Geometry: final body of the model. Coordinates: model frame, mm. Give positions to 0.01 mm unless a question says otherwise; leave off trailing zeros. Write each loop counter-clockwise with the first axis right and the second up, starting at its lowest first coordinate (ties: lowest second). Pieces come first, ordered by that corner, then holes. Notation, with made-up numbers: M -17,7 L 32,7 A26 cw 32,36 Z; hole C -37.5,45.25 d7. An arc over 180 degrees is marked long. Use a Markdown table: item, result. Add a question column.
(1) Draft query along Z for faces 1 (the flat face through (11, 25, 127)), 2 (the flat face through (12, 50.8, 2)), 3 (the cylindrical face through (825.44, 25.04, -2.79)). Return one class per face: released by +Z, released by -Z, zero draft, split by the parting line, or undercut.
(2) Cut plane D-D (z = -90.5). Output: boundary loops of the cut face in (x, y).
(3) Material intervals for L1, parallel to X at y = 22, z = -25.5; L2, parallel to Z at x = -762, y = 34; L3, parallel to X at y = 22, z = 51, sorted ascending.
(4) Cut plane B-B (y = 42). Output: boundary loops of the cut face in (x, z).
(5) Cut plane C-C (z = 79). Output: boundary loops of the cut face in (x, y).
(6) Cut plane A-A (z = 0). Output: boundary loops of the cut face in (x, y), plus the area to 3 significant figures.
(7) Pin query (flat end, axial travel): pin 1 Ø3 at (y, z) = (21.5, 93) entering from +X; pin 2 Ø3 at (y, z) = (21, -89) entering from -X; pin 3 Ø4 at (y, z) = (24, -84.5) entering from +X. Return the tip coordinate at first contact, or that it passes through.
Autodesk Inventor part; units mm, degrees
ref_plane "YZ Plane" through (0, 0, 0) normal (1, 0, 0) x (0, 1, 0)
ref_plane "XZ Plane" through (0, 0, 0) normal (0, 1, 0) x (-1, 0, 0)
ref_plane "XY Plane" through (0, 0, 0) normal (0, 0, 1) x (1, 0, 0)
sketch "Sketch1" plane through (0, 0, 0) normal (0, 1, 0) x (-1, 0, 0)
  line L0 (-762, 127) -> (762, 127)
  line L1 (762, 127) -> (762, -127) construction
  line L2 (762, -127) -> (-762, -127)
  line L3 (-762, -127) -> (-762, 127) construction
  line L4 (-762, 127) -> (762, -127) construction
  line L5 (762, 127) -> (-762, -127) construction
  arc A0 (762, -127) -> (762, 127) centre (762, 0) ccw
  arc A1 (-762, 127) -> (-762, -127) centre (-762, 0) ccw
  circle A2 centre (762, 0) radius 63.5
  circle A3 centre (-762, 0) radius 63.5
  point P0 (0, 0)
  dimension "d0" = 1524
  dimension "d1" = 254
  dimension "d2" = 127
  dimension "d3" = 127
extrude "Extrusion1" add sketch "Sketch1" along normal blind 50.8
properties part number "Output"
Answer list:
| question | item | result |
|---|---|---|
| 1 | face 1 | released by +Z |
| 1 | face 2 | zero draft |
| 1 | face 3 | undercut |
| 2 | outline | M -851.1,0 L 851.1,0 L 851.1,50.8 L -851.1,50.8 Z |
| 3 | L1 | -886.41 to -820.15, -703.85 to 703.85, 820.15 to 886.41 |
| 3 | L2 | -127 to -63.5, 63.5 to 127 |
| 3 | L3 | -878.31 to -799.83, -724.17 to 724.17, 799.83 to 878.31 |
| 4 | outline | M -762,-127 L 762,-127 A127 ccw 762,127 L -762,127 A127 ccw Z; hole C -762,0 d127; hole C 762,0 d127 |
| 5 | outline | M -861.44,0 L 861.44,0 L 861.44,50.8 L -861.44,50.8 Z |
| 6 | outline | M -889,0 L -825.5,0 L -825.5,50.8 L -889,50.8 Z; M -698.5,0 L 698.5,0 L 698.5,50.8 L -698.5,50.8 Z; M 825.5,0 L 889,0 L 889,50.8 L 825.5,50.8 Z |
| 6 | area | 77,400 mm² |
| 7 | pin 1 | x = 850.07 |
| 7 | pin 2 | x = -854.05 |
| 7 | pin 3 | x = 858.55 |
